Geometry check sheet. Reference: the model listing, model coordinates, mm. Face numbers are marked on the shaded views. A direction names the side the tool comes from. Round coordinates to 2 decimals unless told otherwise and drop trailing zeros. Write each loop counter-clockwise with the first axis right and the second up, starting at its lowest first coordinate (ties: lowest second). Pieces come first, ordered by that corner, then holes.
Item 1: Access from +Z, -Z, +X, -X, +Y, -Y to the whole of each face (thin tool, end or side, straight path). Record for the marked faces 5, 6 and 7.
Item 2: Depth check by flat-ended pin: P1, Ø8, axis at x = -21, y = -74.5, coming from the -Z side; P2, Ø23.5, axis at x = -73, y = -42.5, coming from the +Z side; P3, Ø4, axis at y = -45.5, z = 68.5, coming from the -X side. Enter the tip coordinate at first touch or a pass-through.
Item 3: Cross-section at B-B (y = -37). Enter the section's corners in (x, z).
Item 4: Scan lines: probe 1 along Y at (x, z) = (-41.5, 33); probe 2 along Y at (x, z) = (-70.5, 32.5); probe 3 along Z at (x, y) = (-48.5, -67.5). Record each from-to range of solid material in increasing order.
Item 5: Draft check along Y on the marked faces 1, 2, 3 and 4. Enter one of: pulls with the +Y half, pulls with the -Y half, needs draft (parallel to the pull), parting line crosses it, or undercut.
Item 6: Cross-section at A-A (z = 36). Enter the section's corners in (x, y).
Item 7: Cross-section at D-D (y = -48). Enter the section's corners in (x, z), then the cut area to 3 significant figures.
Item 8: Cross-section at C-C (x = -32). Enter the section's corners in (y, z), then the cut area to 3 significant figures.
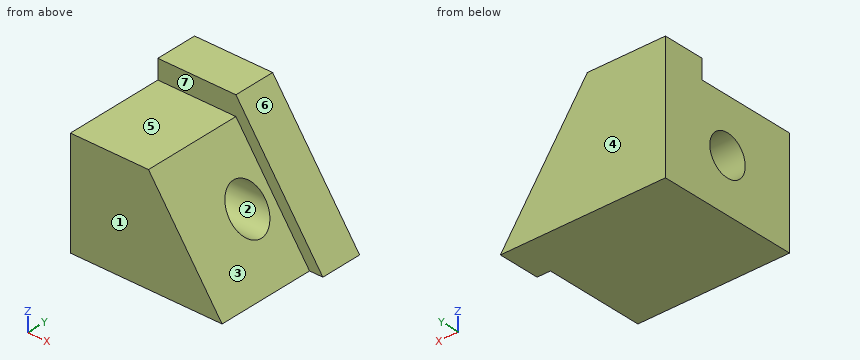
from build123d import *

# Parameters (mm, degrees)
F1_DEPTH = 85.852
F3_DEPTH = 25.4
F4_R     = 12.233243
F5_DEPTH = 100.197954


with BuildPart() as f1:
    # F0 (on Front) → F1 (new body)
    with BuildSketch(Plane.XZ):
        Polygon((-92.0972, 0), (0, 0), (-44.692129, 64.682215), (-92.0972, 64.682215), align=None)
    extrude(amount=F1_DEPTH)

    # F2 (on face) → F3 (join)
    with BuildSketch(Plane(origin=(0, 0, 0), x_dir=(-1, 0, 0), z_dir=(0, 1, 0))):
        Polygon((44.692129, 64.682215), (92.0972, 64.682215), (92.0972, 76.404862), (44.692129, 76.404862), (-8.099754, 0), (0, 0), align=None)
    extrude(amount=-F3_DEPTH)

    # F4 (on face) → F5 (cut, through all)
    with BuildSketch(Plane(origin=(-92.0972, 0, 0), x_dir=(0, -1, 0), z_dir=(-1, 0, 0))):
        with Locations((42.926, 32.341108)):
            Circle(F4_R)
    extrude(amount=-F5_DEPTH, mode=Mode.SUBTRACT)


solid = f1.part
Resolved:
1. face 5: +Z, +X, -X, -Y
1. face 6: +Z, +X, +Y, -Y
1. face 7: +Z, +X, -Y
2. P1: stops at z = 0
2. P2: stops at z = 64.68
2. P3: passes through
3. outline: (-92.1, 0) - (0, 0) - (-14.95, 21.64) - (-92.1, 21.64) - close; (-92.1, 43.04) - (-29.74, 43.04) - (-44.69, 64.68) - (-92.1, 64.68) - close
4. probe 1: y = -85.85 to -55.14, -30.71 to 0
4. probe 2: y = -85.85 to -55.16, -30.69 to 0
4. probe 3: z = 0 to 64.68
5. face 1: pulls with the -Y half
5. face 2: undercut
5. face 3: needs draft
5. face 4: pulls with the +Y half
6. outline: (-92.1, -85.85) - (-24.87, -85.85) - (-24.87, -54.6) - (-92.1, -54.6) - close; (-92.1, -31.25) - (-24.87, -31.25) - (-24.87, -25.4) - (-16.77, -25.4) - (-16.77, 0) - (-92.1, 0) - close
7. outline: (-92.1, 0) - (0, 0) - (-14.65, 21.21) - (-92.1, 21.21) - close; (-92.1, 43.47) - (-30.04, 43.47) - (-44.69, 64.68) - (-92.1, 64.68) - close
7. area: 2,960 mm2
8. outline: (-85.85, 0) - (0, 0) - (0, 58.04) - (-25.4, 58.04) - (-25.4, 46.31) - (-85.85, 46.31) - close; hole circle Ø24.47 at (-42.93, 32.34)
8. area: 3,800 mm2
